from build123d import *

# Parameters (mm, degrees)
SKETCH1_W           = 42.3
SKETCH1_H           = 3.75
BOSS_EXTRUDE1_DEPTH = 15
FILLET1_R           = 0.8255


with BuildPart() as part:
    # Sketch1 → Boss-Extrude1 (new body)
    with BuildSketch(Plane.XY):
        with BuildLine():
            Line((21.15, 0), (21.15, 20.111200005))
            ThreePointArc((21.15, 20.111200005), (20.489653579, 25.354919699), (18.549849056, 30.271200005))
            Line((18.549849056, 30.271200005), (13.550249835, 30.271200005))
            ThreePointArc((13.550249835, 30.271200005), (0, 3.175), (-13.550249835, 30.271200005))
            Line((-13.550249835, 30.271200005), (-18.549849056, 30.271200005))
            ThreePointArc((-18.549849056, 30.271200005), (-20.489653579, 25.354919699), (-21.15, 20.111200005))
            Line((-21.15, 20.111200005), (-21.15, 0))
            Line((-21.15, 0), (21.15, 0))
        make_face()
        with Locations((0, -1.875)):
            Rectangle(SKETCH1_W, SKETCH1_H)
    extrude(amount=BOSS_EXTRUDE1_DEPTH)

    # Fillet1
    fillet1_edges = [part.edges().sort_by_distance(p)[0] for p in [
        (-18.549849056, 30.271200005, 7.5),
        (-13.550249835, 30.271200005, 7.5),
        (13.550249835, 30.271200005, 7.5),
        (18.549849056, 30.271200005, 7.5),
    ]]
    fillet(fillet1_edges, radius=FILLET1_R)


solid = part.part
Design review of the part built by this model. Coordinates are the model's own, in mm. A direction names the side the tool comes from. Coordinates: 2 decimals unless noted, no trailing zeros. Order: outer loops, then holes, each group sorted by start corner. A loop starts at its lowest first (then second) coordinate and runs counter-clockwise, first axis right, second up. Notation, with made-up numbers: (-1.5, 12) -> (37.5, 12) arc R10 ccw to (37.5, 18) -> close; hole circle Ø9 at (72.25, -38.5). An arc over 180 degrees is marked (long way). Use one line per item in the form item = value. Start each with the question number.
(1) Add section D-D on x = 0. State the section outline as (y, z) points (3 decimals), plus the area to 3 significant figures.
(2) Add section B-B on z = 5.5. State the section outline as (x, y) points.
(3) The part is to be moulded in two halves that separate along Y. For faces 3 (the flat face through (21.15, 8, 7)), 4 (the cylindrical face through (0.504, 3.182, 7.395)), 5 (the cylindrical face through (20.567, 25.041, 7.395)), say which applies: +Y half, -Y half, draft (parallel to the pull), parting line (faces both ways), or undercut.
(4) Add section A-A on y = 15.5. State the section outline as (x, z) points, plus the area to 3 significant figures.
(5) For faces 1 (the cylindrical face through (14.396, 29.858, 7.605)), 2 (the cylindrical face through (-20.534, 25.178, 7.395)), list the 3-axis set-ups (+Z, -Z, +X, -X, +Y, -Y) from which the entire face can be reached by the end or side of a thin tool; tool diameter is ignored.
(6) Add section C-C on y = 8. State the section outline as (x, z) points, plus the area to 3 significant figures.
(7) For probe 1 along X at (y, z) = (11, 11); probe 2 along X at (y, z) = (20, 11.5); probe 3 along Y at (x, z) = (0, 5) (3 decimals), list the stretches that pass through material, from the lowest coordinate up.
Answer block:
q1.outline = (-3.75, 0) -> (3.175, 0) -> (3.175, 15) -> (-3.75, 15) -> close
q1.area = 104 mm²
q2.outline = (-21.15, -3.75) -> (21.15, -3.75) -> (21.15, 20.11) arc R21.15 ccw to (18.79, 29.82) arc R0.83 ccw to (18.05, 30.27) -> (15.11, 30.27) arc R0.83 ccw to (14.41, 29.01) arc R16.94 cw (long way) to (-14.41, 29.01) arc R0.83 ccw to (-15.11, 30.27) -> (-18.05, 30.27) arc R0.83 ccw to (-18.79, 29.82) arc R21.15 ccw to (-21.15, 20.11) -> close
q3.face_3 = draft
q3.face_4 = undercut
q3.face_5 = +Y half
q4.outline = (-21.15, 0) -> (-16.3, 0) -> (-16.3, 15) -> (-21.15, 15) -> close; (16.3, 0) -> (21.15, 0) -> (21.15, 15) -> (16.3, 15) -> close
q4.area = 146 mm²
q5.face_1 = +Z, -Z
q5.face_2 = +Z, -Z, -X, +Y
q6.outline = (-21.15, 0) -> (-11.84, 0) -> (-11.84, 15) -> (-21.15, 15) -> close; (11.84, 0) -> (21.15, 0) -> (21.15, 15) -> (11.84, 15) -> close
q6.area = 279 mm²
q7.probe_1 = -21.15 to -14.28, 14.28 to 21.15
q7.probe_2 = -21.15 to -16.94, 16.94 to 21.15
q7.probe_3 = -3.75 to 3.175
